from build123d import *

# Parameters (mm, degrees)
SKETCH1_W           = 279.4
SKETCH1_H           = 254
BOSS_EXTRUDE1_DEPTH = 4.800000052
SKETCH4_W           = 13.148347957
SKETCH4_H           = 12.442555781
SKETCH4_W_2         = 3.81
SKETCH4_H_2         = 12.7
SKETCH4_W_3         = 12.512633495
CUT_EXTRUDE1_DEPTH  = 378.628653575
FILLET1_R           = 6.35


with BuildPart() as part:
    # Sketch1 → Boss-Extrude1 (new body)
    with BuildSketch(Plane.XY):
        with Locations((139.7, 127)):
            Rectangle(SKETCH1_W, SKETCH1_H)
    extrude(amount=BOSS_EXTRUDE1_DEPTH)

    # Sketch4 → Cut-Extrude1 (cut, through all)
    with BuildSketch(Plane(origin=(0, 0, 0), x_dir=(-1, 0, 0), z_dir=(0, 0, -1))):
        Polygon((0, 0), (0, 72.835400266), (-18.411229684, 72.724077305), (-88.95741747, 143.27026509), (-105.001094941, 143.27026509), (-117.513728436, 143.27026509), (-161.28323771, 143.27026509), (-174.431585667, 143.27026509), (-190.55741747, 143.27026509), (-260.35, 73.47768256), (-279.4, 73.47768256), (-279.4, 0), align=None)
        Polygon((-88.9, 168.72768256), (0, 79.82768256), (0, 254), (-279.4, 254), (-279.4, 79.82768256), (-190.5, 168.72768256), align=None)
        with Locations((-167.857411689, 149.491542981)):
            Rectangle(SKETCH4_W, SKETCH4_H)
        with Locations((-139.75741747, 156.02768256)):
            Rectangle(SKETCH4_W_2, SKETCH4_H_2)
        with Locations((-111.257411689, 149.491542981)):
            Rectangle(SKETCH4_W_3, SKETCH4_H)
    extrude(amount=-CUT_EXTRUDE1_DEPTH, mode=Mode.SUBTRACT)

    # Fillet1
    # the kernel refuses this fillet: 6.35 mm, written as the material it takes off along each edge
    with BuildSketch(Plane(origin=(105.001094941, 143.27026509, -15.875), x_dir=(0, 1, 0), z_dir=(0, 0, 1)), Plane(origin=(279.4, 73.47768256, -15.875), x_dir=(0, 1, 0), z_dir=(0, 0, 1)), Plane(origin=(174.431585667, 143.27026509, -15.875), x_dir=(1, 0, 0), z_dir=(0, 0, 1)), Plane(origin=(161.28323771, 143.27026509, -15.875), x_dir=(0, 1, 0), z_dir=(0, 0, 1)), Plane(origin=(117.513728436, 143.27026509, -15.875), x_dir=(1, 0, 0), z_dir=(0, 0, 1))) as fillet1_piece_1:
        with BuildLine():
            CenterArc((FILLET1_R, FILLET1_R), FILLET1_R, 180, 90)
            Line((0, FILLET1_R), (0, 0))
            Line((0, 0), (FILLET1_R, 0))
        make_face()
    extrude(amount=36.550000052, mode=Mode.SUBTRACT)
    with BuildSketch(Plane(origin=(18.411229684, 72.724077305, -6.631938595), x_dir=(-0.9999817205970539, 0.006046360207229539, 0), z_dir=(0, 0, 1))) as fillet1_piece_2:
        with BuildLine():
            CenterArc((FILLET1_R * 0.41775991148, -FILLET1_R), FILLET1_R, 90, 45.346433032)
            Line((-FILLET1_R * 0.293609366521, -FILLET1_R * 0.297181566607), (0, 0))
            Line((0, 0), (FILLET1_R * 0.41775991148, 0))
        make_face()
    extrude(amount=18.063877241, mode=Mode.SUBTRACT)
    with BuildSketch(Plane(origin=(0, 72.835400266, -15.779302468), x_dir=(0, 1, 0), z_dir=(0, 0, 1))) as fillet1_piece_3:
        with BuildLine():
            CenterArc((FILLET1_R * 0.993971809004, -FILLET1_R), FILLET1_R, 90, 89.653566968)
            Line((-FILLET1_R * 0.00600991159307, -FILLET1_R * 0.993953639793), (0, 0))
            Line((0, 0), (FILLET1_R * 0.993971809004, 0))
        make_face()
    extrude(amount=36.358604988, mode=Mode.SUBTRACT)
    with BuildSketch(Plane(origin=(260.35, 73.47768256, -6.575640303), x_dir=(1, 0, 0), z_dir=(0, 0, 1)), Plane(origin=(190.5, 168.72768256, -6.575640303), x_dir=(-1, 0, 0), z_dir=(0, 0, 1)), Plane(origin=(279.4, 79.82768256, -6.575640303), x_dir=(-0.7071067811865475, 0.7071067811865475, 0), z_dir=(0, 0, 1)), Plane(origin=(0, 79.82768256, -6.575640303), x_dir=(0, -1, 0), z_dir=(0, 0, 1)), Plane(origin=(88.9, 168.72768256, -6.575640303), x_dir=(-0.7071067811865476, -0.7071067811865476, 0), z_dir=(0, 0, 1))) as fillet1_piece_4:
        with BuildLine():
            CenterArc((FILLET1_R * 0.414213562373, FILLET1_R), FILLET1_R, 225, 45)
            Line((-FILLET1_R * 0.292893218813, FILLET1_R * 0.292893218813), (0, 0))
            Line((0, 0), (FILLET1_R * 0.414213562373, 0))
        make_face()
    extrude(amount=17.951280657, mode=Mode.SUBTRACT)


solid = part.part
The listing builds one solid part. Answer for the finished solid, in the listing's coordinates (mm). A direction names the side the tool comes from. Give positions to 0.01 mm unless a question says otherwise; leave off trailing zeros. Order: outer loops, then holes, each group sorted by start corner. A loop starts at its lowest first (then second) coordinate and runs counter-clockwise, first axis right, second up. Notation, with made-up numbers: (78, 61) - (124, 61) arc R20 cw to (124, 89) - close; hole circle Ø3 at (-32.5, 28.25). An arc over 180 degrees is marked (long way). Answer as CSV lines item,"result".
Q1. Determine the mould class of faces 1 (the face through (190.33, 168.23, 2.37)), 2 (the face through (94, 143.27, 2)), 3 (the face through (140, 168.728, 2)) for opening direction X: pulls with the +X half, pulls with the -X half, needs draft (parallel to the pull), parting line crosses it, or undercut.
Answer key:
face 1,"pulls with the +X half"
face 2,"undercut"
face 3,"needs draft"
Q2. A cutting plane is placed at C-C, the plane x = 177. Determine the outline of the cut face in (y, z), and give its area (3 significant figures).
Answer key:
outline,"(144.52, 0) - (168.73, 0) - (168.73, 4.8) - (144.52, 4.8) - close"
area,"116 mm^2"
Q3. A cutting plane is placed at D-D, the plane x = 129. Determine the outline of the cut face in (y, z).
Answer key:
outline,"(143.27, 0) - (168.73, 0) - (168.73, 4.8) - (143.27, 4.8) - close"
Q4. A cutting plane is placed at B-B, the plane y = 85. Determine the outline of the cut face in (x, z).
Answer key:
outline,"(5.17, 0) - (30.69, 0) - (30.69, 4.8) - (5.17, 4.8) - close; (248.83, 0) - (274.23, 0) - (274.23, 4.8) - (248.83, 4.8) - close"
Q5. Straight lines are drawn through the part: L1, parallel to X at y = 151.5, z = 3.45; L2, parallel to X at y = 109, z = 4.25; L3, parallel to X at y = 135.5, z = 1.35. For each, find the intervals that lie inside material, in ascending order.
Answer key:
L1,"x = 71.67 to 105, 117.51 to 137.85, 141.66 to 161.28, 174.43 to 207.73"
L2,"x = 29.17 to 54.69, 224.83 to 250.23"
L3,"x = 55.67 to 81.19, 198.33 to 223.73"
Q6. Which of the six approach directions +Z, -Z, +X, -X, +Y, -Y give full straight-line access (tool end or side, diameter ignored) to faces 4 (the face through (235.55, 123.68, 2.37)), 5 (the face through (141.662, 156, 2)), 6 (the face through (18.177, 73.203, 2.366))?
Answer key:
face 4,"+Z, -Z, +X, +Y"
face 5,"+Z, -Z"
face 6,"+Z, -Z, -Y"
Q7. Each of these flat-tipped pins is pushed along its axis until it touches: pin 1 Ø1.9 at (x, z) = (139.5, 2) entering from -Y; pin 2 Ø1.4 at (y, z) = (151.5, 1.5) entering from -X; pin 3 Ø2.5 at (y, z) = (158.5, 3) entering from -X. Where does it stop, or does it pass through?
Answer key:
pin 1,"stops at y = 143.27"
pin 2,"stops at x = 70.97"
pin 3,"stops at x = 77.42"
